```python
from build123d import *

# Parameters (mm, degrees)
F0_W     = 76.2
F0_H     = 75.435378
F0_R     = 16.244166
F0_H_2   = 70.614622
F0_W_2   = 25.4
F0_H_3   = 25.4
F1_DEPTH = 19.05


with BuildPart() as f1:
    # F0 (on Front) → F1 (new body)
    with BuildSketch(Plane.XZ):
        with Locations((-38.1, 37.717689)):
            Rectangle(F0_W, F0_H)
        with Locations((-38.1, 39.470069)):
            Circle(F0_R, mode=Mode.SUBTRACT)
        with Locations((-38.1, 110.742689)):
            Rectangle(F0_W, F0_H_2)
        with Locations((-38.1, 109.5248)):
            Rectangle(F0_W_2, F0_H_3, mode=Mode.SUBTRACT)
    extrude(amount=F1_DEPTH)


solid = f1.part
```
Input: part model. Units: mm. Frame: model coordinates. A direction names the side the tool comes from. Give positions to 0.01 mm unless a question says otherwise; leave off trailing zeros. Write each loop counter-clockwise with the first axis right and the second up, starting at its lowest first coordinate (ties: lowest second). Pieces come first, ordered by that corner, then holes. Notation, with made-up numbers: (65.25, 46) - (99.25, 46) arc R17 ccw to (99.25, 69) - close; hole circle Ø8 at (73.5, -2.75). An arc over 180 degrees is marked (long way). Write item = value, one per line. Start each with the question number.
1. Access query for faces 1 (the flat face through (-25.4, -9, 109)), 2 (the flat face through (-39, 0, 74)). Directions: +Z, -Z, +X, -X, +Y, -Y. A direction counts if a zero-diameter tool reaches every point of the face in a straight line with its end or side. Return the directions, or none.
2. Section query A-A, the plane x = -38.1. Output: boundary loops of the cut face in (y, z).
3. Mould query, pull axis X, two halves, no side actions, for faces 3 (the flat face through (-50.8, -9, 109)), 4 (the flat face through (0, -9, 72)), 5 (the flat face through (-39, -19.05, 74)), 6 (the flat face through (-76.2, -9, 74)). Classes: released by +X, released by -X, zero draft, split by the parting line, or undercut.
4. Ray query, L1, parallel to Z at x = -38.1, y = -13.5; L2, parallel to X at y = -7, z = 118.5; L3, parallel to Z at x = -26.5, y = -15. Return the intervals inside material, ascending.
5. Section query B-B, the plane y = -10.5. Output: boundary loops of the cut face in (x, z), then the cut area to 3 significant figures.
6. First-contact query: pin 1 Ø19.5 at (x, z) = (-38.1, 39.47) entering from +Y. Flat tip, straight axial feed; report the tip coordinate or a pass-through.
Check sheet entries:
q1.face_1 = +Y, -Y
q1.face_2 = +Z, -Z, +X, -X, +Y
q2.outline = (-19.05, 0) - (0, 0) - (0, 23.23) - (-19.05, 23.23) - close; (-19.05, 55.71) - (0, 55.71) - (0, 96.82) - (-19.05, 96.82) - close; (-19.05, 122.22) - (0, 122.22) - (0, 146.05) - (-19.05, 146.05) - close
q3.face_3 = undercut
q3.face_4 = released by +X
q3.face_5 = zero draft
q3.face_6 = released by -X
q4.L1 = 0 to 23.23, 55.71 to 96.82, 122.22 to 146.05
q4.L2 = -76.2 to -50.8, -25.4 to 0
q4.L3 = 0 to 28.1, 50.84 to 96.82, 122.22 to 146.05
q5.outline = (-76.2, 0) - (0, 0) - (0, 146.05) - (-76.2, 146.05) - close; hole circle Ø32.49 at (-38.1, 39.47); hole (-50.8, 96.82) - (-25.4, 96.82) - (-25.4, 122.22) - (-50.8, 122.22) - close
q5.area = 9,650 mm2
q6.pin_1 = through
